from build123d import *

# Parameters (mm, degrees)
SALIENTE_EXTRUIR1_DEPTH = 1
SALIENTE_EXTRUIR2_DEPTH = 1


with BuildPart() as part:
    # Croquis1 → Saliente-Extruir1 (new body)
    with BuildSketch(Plane.XY):
        with BuildLine():
            Line((-77.34358908, -6.813189194), (-77.34358908, 0.186810806))
            ThreePointArc((-77.34358908, 0.186810806), (-74.44358908, 3.086810806), (-71.54358908, 0.186810806))
            Line((-71.54358908, 0.186810806), (-71.54358908, -6.813189194))
            Line((-71.54358908, -6.813189194), (-71.54358908, -7.813189194))
            Line((-71.54358908, -7.813189194), (-70.54358908, -7.813189194))
            Line((-70.54358908, -7.813189194), (-70.54358908, 0.185713536))
            ThreePointArc((-70.54358908, 0.185713536), (-74.44358908, 4.085713536), (-78.34358908, 0.185713536))
            Line((-78.34358908, 0.185713536), (-78.34358908, -7.813189194))
            Line((-78.34358908, -7.813189194), (-77.34358908, -7.813189194))
            Line((-77.34358908, -7.813189194), (-77.34358908, -6.813189194))
        make_face()
    extrude(amount=SALIENTE_EXTRUIR1_DEPTH)

    # Croquis3 → Saliente-Extruir2 (add)
    with BuildSketch(Plane.XY.offset(1)):
        with BuildLine():
            Line((-77.34358908, -7.813189194), (-78.34358908, -7.813189194))
            Line((-78.34358908, -7.813189194), (-78.34358908, 0.185713536))
            ThreePointArc((-78.34358908, 0.185713536), (-74.44358908, 4.085713536), (-70.54358908, 0.185713536))
            Line((-70.54358908, 0.185713536), (-70.54358908, -7.813189194))
            Line((-70.54358908, -7.813189194), (-77.34358908, -7.813189194))
        make_face()
    extrude(amount=SALIENTE_EXTRUIR2_DEPTH)


solid = part.part
Build history of the part. All positions in model axes, mm. A direction names the side the tool comes from. Coordinates: 2 decimals unless noted, no trailing zeros. Write each loop counter-clockwise with the first axis right and the second up, starting at its lowest first coordinate (ties: lowest second). Pieces come first, ordered by that corner, then holes.
(1) Pin check, flat tip, straight feed: pin 1 Ø1 at (x, y) = (-76.5, -5) entering from -Z. Stop position of the tip, or through.
(2) Drill centre lines: line 1 (X direction, y = 0, z = 0.8); line 2 (Z direction, x = -76.25, y = -3.75); line 3 (X direction, y = 3.25, z = 1.75). Where is each one in solid material? Low to high.
(3) Mould opens along X. For faces 3 (the cylindrical face through (-74.507, 3.086, 0.493)), 4 (the flat face through (-70.544, -4, 1)), 5 (the flat face through (-78, -1, 0)), 6 (the flat face through (-78.344, -4, 1)) say: pulls with the +X half, pulls with the -X half, needs draft (parallel to the pull), parting line crosses it, or undercut.
(4) Cut at C-C on x = -72. List the corners of the cut face in (y, z), and give its area (3 significant figures).
(5) Cut at D-D on z = 1.5. List the corners of the cut face in (x, y), and give its area (3 significant figures).
(6) Cut at B-B on z = 0.5. List the corners of the cut face in (x, y).
(7) Cut at A-A on y = -1. List the corners of the cut face in (x, z), and give its area (3 significant figures).
(8) 3-axis set-ups, long thin cutter, end or side, ignore diameter. For faces 1 (the flat face through (-77.344, -3.9, 0.5)), 2 (the flat face through (-74.4, -7.813, 1.4)): which of +Z, -Z, +X, -X, +Y, -Y reach the whole face in a straight line?
Working result:
1. pin 1: stops at z = 1
2. line 1: x = -78.34 to -77.34, -71.54 to -70.54
2. line 2: z = 1 to 2
2. line 3: x = -76.86 to -72.03
3. face 3: undercut
3. face 4: pulls with the +X half
3. face 5: needs draft
3. face 6: pulls with the -X half
4. outline: (-7.81, 1) - (1.75, 1) - (1.75, 0) - (3.23, 0) - (3.23, 2) - (-7.81, 2) - close
4. area: 12.5 mm2
5. outline: (-78.34, -7.81) - (-70.54, -7.81) - (-70.54, 0.19) arc R3.9 ccw to (-78.34, 0.19) - close
5. area: 86.3 mm2
6. outline: (-78.34, -7.81) - (-77.34, -7.81) - (-77.34, 0.19) arc R2.9 cw to (-71.54, 0.19) - (-71.54, -7.81) - (-70.54, -7.81) - (-70.54, 0.19) arc R3.9 ccw to (-78.34, 0.19) - close
7. outline: (-78.34, 0) - (-77.34, 0) - (-77.34, 1) - (-71.54, 1) - (-71.54, 0) - (-70.54, 0) - (-70.54, 2) - (-78.34, 2) - close
7. area: 9.80 mm2
8. face 1: -Z, -Y
8. face 2: +Z, -Z, +X, -X, -Y
